Geometry: final body of the model. Coordinates: model frame, mm. Face numbers are marked on the shaded views. Coordinates: 2 decimals unless noted, no trailing zeros. Order: outer loops, then holes, each group sorted by start corner. A loop starts at its lowest first (then second) coordinate and runs counter-clockwise, first axis right, second up. Notation, with made-up numbers: M -26.5,51.25 L 9.5,51.25 A11 cw 9.5,58.25 Z; hole C -14,59 d10. An arc over 180 degrees is marked long. Write item = value, one per line. Start each with the question number.
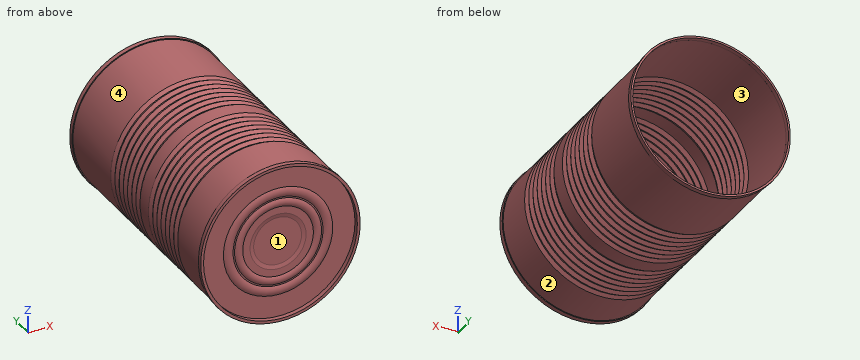
```python
from build123d import *


with BuildPart() as part:
    # Sketch1 → Revolve1 (revolve)
    with BuildSketch(Plane.XY):
        with BuildLine():
            Line((0, 0), (16.383, 0))
            Line((16.383, 0), (19.177, -0.635))
            Line((19.177, -0.635), (24.1935, -0.635))
            ThreePointArc((24.1935, -0.635), (26.9875, -1.651), (29.7815, -0.635))
            Line((29.7815, -0.635), (30.7975, -0.635))
            ThreePointArc((30.7975, -0.635), (34.0995, -1.651), (37.4015, -0.635))
            Line((37.4015, -0.635), (52.65050938, -0.635))
            Line((52.65050938, -0.635), (52.65050938, -3.81))
            Line((52.65050938, -3.81), (54.58856494, -3.81))
            Line((54.58856494, -3.81), (54.58856494, -0.635))
            Line((54.58856494, -0.635), (53.94254642, -0.635))
            Line((53.94254642, -0.635), (53.94254642, 27.94))
            Line((53.94254642, 27.94), (52.48900475, 30.734))
            Line((52.48900475, 30.734), (53.94254642, 33.528))
            Line((53.94254642, 33.528), (52.48900475, 36.322))
            Line((52.48900475, 36.322), (53.94254642, 39.116))
            Line((53.94254642, 39.116), (52.48900475, 41.91))
            Line((52.48900475, 41.91), (53.94254642, 44.704))
            Line((53.94254642, 44.704), (52.48900475, 47.498))
            Line((52.48900475, 47.498), (53.94254642, 50.292))
            Line((53.94254642, 50.292), (52.48900475, 53.086))
            Line((52.48900475, 53.086), (53.94254642, 55.88))
            Line((53.94254642, 55.88), (52.48900475, 58.674))
            Line((52.48900475, 58.674), (53.94254642, 61.468))
            Line((53.94254642, 61.468), (52.48900475, 64.262))
            Line((52.48900475, 64.262), (53.94254642, 67.056))
            Line((53.94254642, 67.056), (53.94254642, 78.232))
            Line((53.94254642, 78.232), (52.48900475, 81.026))
            Line((52.48900475, 81.026), (53.94254642, 83.82))
            Line((53.94254642, 83.82), (52.48900475, 86.614))
            Line((52.48900475, 86.614), (53.94254642, 89.408))
            Line((53.94254642, 89.408), (52.48900475, 92.202))
            Line((52.48900475, 92.202), (53.94254642, 94.996))
            Line((53.94254642, 94.996), (52.48900475, 97.79))
            Line((52.48900475, 97.79), (53.94254642, 100.584))
            Line((53.94254642, 100.584), (52.48900475, 103.378))
            Line((52.48900475, 103.378), (53.94254642, 106.172))
            Line((53.94254642, 106.172), (52.48900475, 108.966))
            Line((52.48900475, 108.966), (53.94254642, 111.76))
            Line((53.94254642, 111.76), (52.48900475, 114.554))
            Line((52.48900475, 114.554), (53.94254642, 117.348))
            Line((53.94254642, 117.348), (53.94254642, 167.64))
            Line((53.94254642, 167.64), (54.58856494, 167.64))
            Line((54.58856494, 167.64), (54.58856494, 170.815))
            Line((54.58856494, 170.815), (53.31856494, 170.815))
            Line((53.31856494, 170.815), (53.31856494, 167.64))
            Line((53.31856494, 167.64), (53.30754642, 167.64))
            Line((53.30754642, 167.64), (53.30754642, 117.503296069))
            Line((53.30754642, 117.503296069), (51.773214017, 114.554))
            Line((51.773214017, 114.554), (53.226755687, 111.76))
            Line((53.226755687, 111.76), (51.773214017, 108.966))
            Line((51.773214017, 108.966), (53.226755687, 106.172))
            Line((53.226755687, 106.172), (51.773214017, 103.378))
            Line((51.773214017, 103.378), (53.226755687, 100.584))
            Line((53.226755687, 100.584), (51.773214017, 97.79))
            Line((51.773214017, 97.79), (53.226755687, 94.996))
            Line((53.226755687, 94.996), (51.773214017, 92.202))
            Line((51.773214017, 92.202), (53.226755687, 89.408))
            Line((53.226755687, 89.408), (51.773214017, 86.614))
            Line((51.773214017, 86.614), (53.226755687, 83.82))
            Line((53.226755687, 83.82), (51.773214017, 81.026))
            Line((51.773214017, 81.026), (53.30754642, 78.076703931))
            Line((53.30754642, 78.076703931), (53.30754642, 67.211296069))
            Line((53.30754642, 67.211296069), (51.773214017, 64.262))
            Line((51.773214017, 64.262), (53.226755687, 61.468))
            Line((53.226755687, 61.468), (51.773214017, 58.674))
            Line((51.773214017, 58.674), (53.226755687, 55.88))
            Line((53.226755687, 55.88), (51.773214017, 53.086))
            Line((51.773214017, 53.086), (53.226755687, 50.292))
            Line((53.226755687, 50.292), (51.773214017, 47.498))
            Line((51.773214017, 47.498), (53.226755687, 44.704))
            Line((53.226755687, 44.704), (51.773214017, 41.91))
            Line((51.773214017, 41.91), (53.226755687, 39.116))
            Line((53.226755687, 39.116), (51.773214017, 36.322))
            Line((51.773214017, 36.322), (53.226755687, 33.528))
            Line((53.226755687, 33.528), (51.773214017, 30.734))
            Line((51.773214017, 30.734), (53.30754642, 27.784703931))
            Line((53.30754642, 27.784703931), (53.30754642, 0))
            Line((53.30754642, 0), (37.199965126, 0))
            ThreePointArc((37.199965126, 0), (34.0995, -1.016), (30.999034874, 0))
            Line((30.999034874, 0), (29.540168408, 0))
            ThreePointArc((29.540168408, 0), (26.9875, -1.016), (24.434831592, 0))
            Line((24.434831592, 0), (19.2482506, 0))
            Line((19.2482506, 0), (16.4542506, 0.635))
            Line((16.4542506, 0.635), (0, 0.635))
            Line((0, 0.635), (0, 0))
        make_face()
    revolve(axis=Axis((0, -1000, 0), (0, 1, 0)))


solid = part.part
```
Item 1: First-contact query: pin 1 (6 mm diameter, centred on y = 75.5, z = 12.5, fed in from +X); pin 2 (1.5 mm diameter, centred on x = -2, y = 54, fed in from +Z); pin 3 (1 mm diameter, centred on x = 23, y = 49, fed in from -Z). Flat tips, straight axial feed; report the tip coordinate or a pass-through.
Item 2: Draft query along Y for the marked faces 1, 2, 3 and 4. Return one class per face: pulls with the +Y half, pulls with the -Y half, needs draft (parallel to the pull), parting line crosses it, or undercut.
Item 3: Material intervals for probe 1 along Z at (x, y) = (0, -2); probe 2 along Z at (x, y) = (0, 75), sorted ascending. Write a range as [from, to].
Item 4: Section query A-A on y = 150. Output: boundary loops of the cut face in (x, z).
Ans:
q1.pin_1 = 53.1
q1.pin_2 = 53.32
q1.pin_3 = -48.42
q2.face_1 = pulls with the -Y half
q2.face_2 = undercut
q2.face_3 = needs draft
q2.face_4 = undercut
q3.probe_1 = [-54.59, -52.65], [52.65, 54.59]
q3.probe_2 = [-53.94, -53.31], [53.31, 53.94]
q4.outline = C 0,0 d107.89; hole C 0,0 d106.62
